Input: dimensioned drawing with shaded views. Units: mm. Origin: part minimum x, y, z. A direction names the side the tool comes from. Coordinates: 2 decimals unless noted, no trailing zeros. Loops run counter-clockwise (first coordinate to the right, second up) from the corner with the lowest first, then second, coordinate; pieces in that order, holes last.
(1) Section D-D, the plane z = 28.5. Return loops of the section in (x, y).
(2) Set-up query: the marked faces 1 and 2. Return all of +Z, -Z, +X, -X, +Y, -Y with unobstructed straight access to the full face (end or side cutting, diameter ignored); none if empty.
(3) Section A-A, the plane z = 21. Return loops of the section in (x, y), then the cut area to 3 significant figures.
(4) Line query: L1, parallel to Y at x = 5.5, z = 19; L2, parallel to X at y = 36, z = 17. Output: solid intervals per line, ascending.
(5) Section B-B, the plane y = 21. Return loops of the section in (x, z), then the cut area to 3 significant figures.
(6) Contact query for flat-ended pins moving along their axis: P1, Ø10, axis at x = 16.5, y = 11, coming from the +Z side; P2, Ø5, axis at x = 36.5, y = 36.5, coming from the +Z side; P3, Ø10, axis at y = 6.5, z = 5, coming from the -X side; P4, Ø3, axis at x = 15, z = 30, coming from the -Y side. Output: stop coordinate, or through.
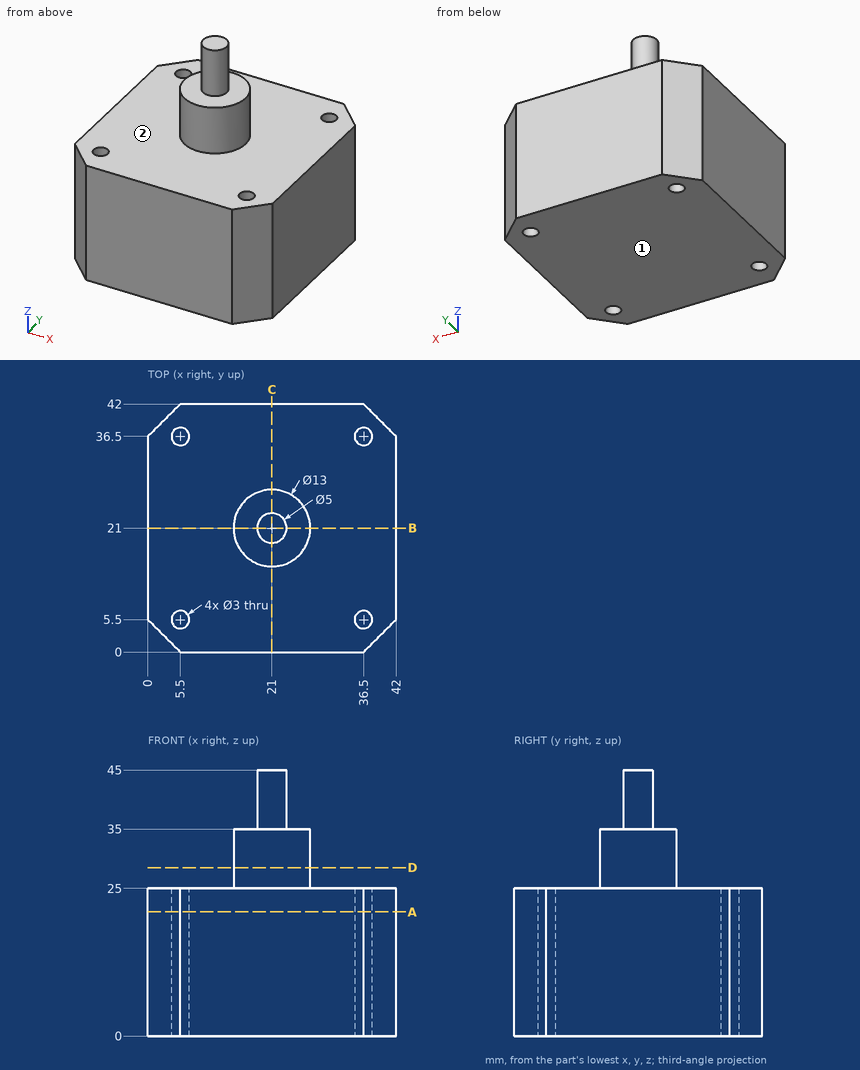
Report:
1. outline: circle Ø13 at (21, 21)
2. face 1: -Z, +X, -X, +Y, -Y
2. face 2: +Z
3. outline: (0, 5.5) - (5.5, 0) - (36.5, 0) - (42, 5.5) - (42, 36.5) - (36.5, 42) - (5.5, 42) - (0, 36.5) - close; hole circle Ø3 at (5.5, 5.5); hole circle Ø3 at (5.5, 36.5); hole circle Ø3 at (36.5, 5.5); hole circle Ø3 at (36.5, 36.5)
3. area: 1,680 mm2
4. L1: y = 0 to 4, 7 to 35, 38 to 42
4. L2: x = 0 to 4.09, 6.91 to 35.09, 37.91 to 42
5. outline: (0, 0) - (42, 0) - (42, 25) - (27.5, 25) - (27.5, 35) - (23.5, 35) - (23.5, 45) - (18.5, 45) - (18.5, 35) - (14.5, 35) - (14.5, 25) - (0, 25) - close
5. area: 1,230 mm2
6. P1: stops at z = 35
6. P2: stops at z = 25
6. P3: stops at x = 0
6. P4: stops at y = 16.31
